Read the model definition and answer for the solid it produces. Units are mm, in the model's axes. Round coordinates to 2 decimals unless told otherwise and drop trailing zeros. Order: outer loops, then holes, each group sorted by start corner. A loop starts at its lowest first (then second) coordinate and runs counter-clockwise, first axis right, second up. Notation, with made-up numbers: (-16, 72) -> (30, 72) arc R20 cw to (30, 92) -> close; hole circle Ø1 at (76.5, 85.25). An arc over 180 degrees is marked (long way). One line per item, written item: value. Start each with the question number.
1. Section C-C (y = 56) is taken. Give the vertices of the cut face in (x, z), then the cut area to 3 significant figures.
2. Section D-D (x = 141.5) is taken. Give the vertices of the cut face in (y, z).
3. Section B-B (x = 20) is taken. Give the vertices of the cut face in (y, z), then the cut area to 3 significant figures.
4. Flat-ended cylindrical pins translate along their axes: pin 1 Ø1 at (x, z) = (32, 0.5) entering from +Y; pin 2 Ø3 at (x, z) = (197.5, 4) entering from +Y; pin 3 Ø14.5 at (x, y) = (20, 20) entering from -Z; pin 4 Ø1 at (x, z) = (146.5, 3) entering from +Y. Find the tip coordinate at first contact, or state that the pin passes through.
5. Section A-A (z = 1.9) is taken. Give the vertices of the cut face in (x, y), then the cut area to 3 significant figures.
6. Consider line 1 (Y direction, x = 20, z = 4.5); line 2 (X direction, y = 15.5, z = 0.8); line 3 (Y direction, x = 87, z = 1.2). Determine where each line is inside the solid, lowest interval first.
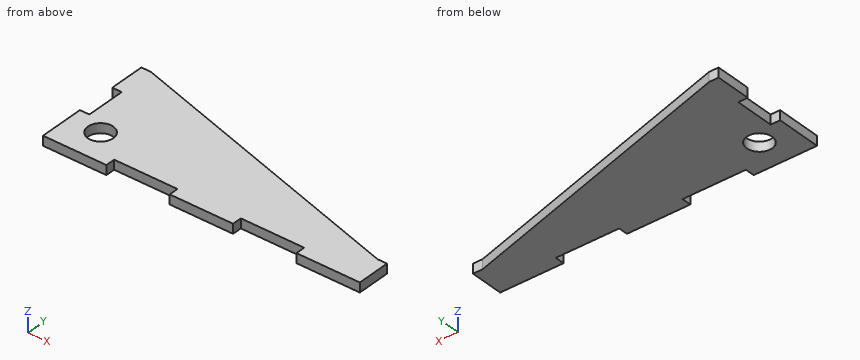
Autodesk Inventor part; units mm, degrees
ref_plane "YZ Plane" through (0, 0, 0) normal (1, 0, 0) x (0, 1, 0)
ref_plane "XZ Plane" through (0, 0, 0) normal (0, 1, 0) x (-1, 0, 0)
ref_plane "XY Plane" through (0, 0, 0) normal (0, 0, 1) x (1, 0, 0)
ref_plane "Work Plane1" through (0, 0, 0) normal (0, 0, 1) x (1, 0, 0)
sketch "Sketch1" plane through (0, 0, 0) normal (0, 0, 1) x (1, 0, 0)
  line L0 (0, 6) -> (40, 6)
  line L1 (0, 0) -> (0, 6)
  line L2 (40, 0) -> (0, 0)
  line L3 (40, 0) -> (40, 6)
  line L4 (80, 0) -> (80, 6)
  line L5 (80, 6) -> (40, 6)
  line L6 (40, 6) -> (40, 0)
  line L7 (40, 0) -> (80, 0)
  line L8 (80, 6) -> (120, 6)
  line L9 (80, 0) -> (80, 6)
  line L10 (120, 0) -> (80, 0)
  line L11 (120, 0) -> (120, 6)
  line L12 (160, 0) -> (160, 6)
  line L13 (160, 6) -> (120, 6)
  line L14 (120, 6) -> (120, 0)
  line L15 (120, 0) -> (160, 0)
  line L16 (160, 6) -> (200, 6)
  line L17 (160, 0) -> (160, 6)
  line L18 (200, 0) -> (160, 0)
  line L19 (200, 6) -> (200, 0)
  line L20 (200, 6) -> (200, 21)
  line L21 (194, 21) -> (200, 21)
  line L22 (194, 21) -> (194, 6)
  line L23 (194, 6) -> (200, 6)
  line L24 (6, 28.5) -> (0, 28.5)
  line L25 (0, 28.5) -> (0, 6)
  line L26 (6, 6) -> (0, 6)
  line L27 (6, 6) -> (6, 28.5)
  line L28 (0, 53.5) -> (0, 28.5)
  line L29 (6, 28.5) -> (0, 28.5)
  line L30 (6, 28.5) -> (6, 53.5)
  line L31 (6, 53.5) -> (0, 53.5)
  line L32 (6, 53.5) -> (0, 53.5)
  line L33 (6, 53.5) -> (6, 76)
  line L34 (6, 76) -> (0, 76)
  line L35 (0, 76) -> (0, 53.5)
  line L36 (6, 76) -> (194, 21)
extrude "Plate1" add sketch "Sketch1" along normal blind 6 contours L25 L24 L27 L0 | L0 L3 L2 L1 | L27 L30 L33 L36 L22 L16 L13 L8 L5 L0 | L35 L34 L33 L31 | L8 L11 L10 L4 | L16 L19 L18 L12 | L21 L20 L16 L22
sketch "Sketch2" plane through (0, 0, 6) normal (0, 0, 1) x (1, 0, 0)
  line L0 (0, 0) -> (0, 28.5)
  line L1 (40, 0) -> (0, 0)
  line L2 (40, 6) -> (40, 0)
  line L3 (80, 6) -> (40, 6)
  line L4 (80, 0) -> (80, 6)
  line L5 (120, 0) -> (80, 0)
  line L6 (120, 6) -> (120, 0)
  line L7 (160, 6) -> (120, 6)
  line L8 (160, 0) -> (160, 6)
  line L9 (200, 0) -> (160, 0)
  line L10 (200, 21) -> (200, 0)
  line L11 (194, 21) -> (200, 21)
  line L12 (6, 76) -> (194, 21)
  line L13 (0, 76) -> (6, 76)
  line L14 (0, 53.5) -> (0, 76)
  line L15 (6, 53.5) -> (0, 53.5)
  line L16 (6, 28.5) -> (6, 53.5)
  line L17 (0, 28.5) -> (6, 28.5)
  circle A0 centre (20, 20) radius 8
  point P0 (0, 0)
  point P1 (20, 0)
  dimension "d1" = 16
  dimension "d2" = 20
extrude "Cut1" cut sketch "Sketch2" against normal blind 6 contours A0
equation "\"d3\" = Thickness"
equation "\"d0\" = Thickness"
equation "\"BendRadius\" = Thickness"
equation "\"BendReliefWidth\" = Thickness"
equation "\"BendReliefDepth\" = 0.5 * Thickness"
equation "\"CornerReliefSize\" = 4 * Thickness"
equation "\"MinimumRemnant\" = 2 * Thickness"
equation "\"TransitionRadius\" = BendRadius"
equation "\"JacobiRadiusSize\" = BendRadius"
equation "\"GapSize\" = Thickness"
properties part number "zijkant elektrobox voor knop" material "Wood (Birch)"
Answer:
1. outline: (0, 0) -> (74.36, 0) -> (74.36, 6) -> (0, 6) -> close
1. area: 446 mm^2
2. outline: (6, 0) -> (36.36, 0) -> (36.36, 6) -> (6, 6) -> close
3. outline: (0, 0) -> (12, 0) -> (12, 6) -> (0, 6) -> close; (28, 0) -> (71.9, 0) -> (71.9, 6) -> (28, 6) -> close
3. area: 335 mm^2
4. pin 1: y = 68.54
4. pin 2: y = 21
4. pin 3: through
4. pin 4: y = 35.04
5. outline: (0, 0) -> (40, 0) -> (40, 6) -> (80, 6) -> (80, 0) -> (120, 0) -> (120, 6) -> (160, 6) -> (160, 0) -> (200, 0) -> (200, 21) -> (194, 21) -> (6, 76) -> (0, 76) -> (0, 53.5) -> (6, 53.5) -> (6, 28.5) -> (0, 28.5) -> close; hole circle Ø16 at (20, 20)
5. area: 8,870 mm^2
6. line 1: 0 to 12, 28 to 71.9
6. line 2: 0 to 13.39, 26.61 to 200
6. line 3: 0 to 52.3
